Could you check a few things on this model? Use its own coordinates, in mm. Face numbers are marked on the shaded views. Coordinates: 2 decimals unless noted, no trailing zeros. Loops run counter-clockwise (first coordinate to the right, second up) from the corner with the lowest first, then second, coordinate; pieces in that order, holes last. Notation, with made-up numbers: (-9.5, -1.5) - (0.5, -1.5) arc R21 ccw to (0.5, 33.5) - close; hole circle Ø4 at (-25, 59). An arc over 180 degrees is marked (long way). One line per item, written item: value. Start each with the question number.
(1) If I drill on line 1 along X through (y, z) = (-0.7, 0) (3 decimals); line 2 along Z through (x, y) = (0, -0.95) (3 decimals), over which ranges is the centre line in solid material (lowest first)? Write a range as from..to.
(2) If we section it at A-A on z = 0: Write out the boundary of the cut face in (x, y) (3 decimals).
(3) I'm going to push flat-ended pins straight in: P1, Ø1.5, axis at y = -0.5, z = 3, coming from the +X side; P2, Ø2, axis at y = -0.5, z = 8.5, coming from the -X side. Where does each tip first touch, or does it pass through?
(4) If we section it at D-D on y = -1.45: Write out the boundary of the cut face in (x, z) (3 decimals).
(5) If we mould it in two halves opening along X, with no side actions, what happens to the marked faces 1 and 2? For each: pulls with the +X half, pulls with the -X half, needs draft (parallel to the pull), parting line crosses it, or undercut.
(6) If we section it at B-B on x = 0: Write out the boundary of the cut face in (y, z) (3 decimals).
(7) If we section it at C-C on z = 7: Write out the boundary of the cut face in (x, y).
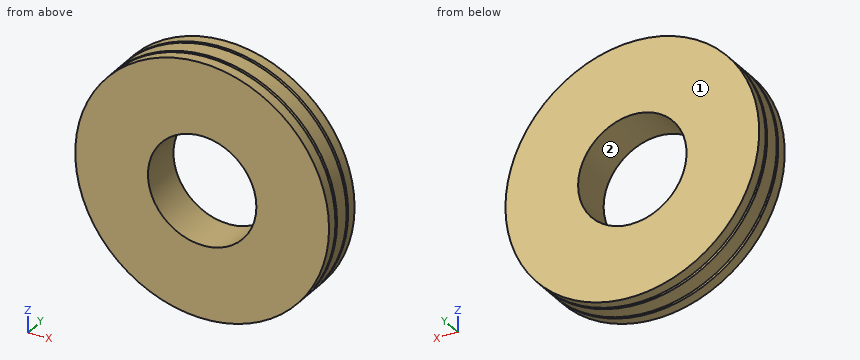
```python
from build123d import *

# Parameters (mm, degrees)
SKETCH1_R           = 11.875
SKETCH1_R_2         = 5.075
BOSS_EXTRUDE1_DEPTH = 2
SKETCH2_R           = 11.875
SKETCH2_R_2         = 11.375
CUT_EXTRUDE1_DEPTH  = 0.25


with BuildPart() as part:
    # Sketch1 → Boss-Extrude1 (new body, symmetric)
    with BuildSketch(Plane(origin=(0, 0, 0), x_dir=(1, 0, 0), z_dir=(0, 1, 0))):
        Circle(SKETCH1_R)
        Circle(SKETCH1_R_2, mode=Mode.SUBTRACT)
    extrude(amount=BOSS_EXTRUDE1_DEPTH, both=True)

    # Sketch2 → Cut-Extrude1 (cut)
    with BuildSketch(Plane(origin=(0, 1, 0), x_dir=(1, 0, 0), z_dir=(0, 1, 0))):
        Circle(SKETCH2_R)
        Circle(SKETCH2_R_2, mode=Mode.SUBTRACT)
    cut_extrude1 = extrude(amount=-CUT_EXTRUDE1_DEPTH, mode=Mode.SUBTRACT)

    # Mirror1: Cut-Extrude1 across plane
    add(cut_extrude1.mirror(Plane.ZX), mode=Mode.SUBTRACT)


solid = part.part
```
Values:
1. line 1: x = -11.875..-5.075, 5.075..11.875
1. line 2: z = -11.375..-5.075, 5.075..11.375
2. outline: (-11.875, -2) - (-5.075, -2) - (-5.075, 2) - (-11.875, 2) - (-11.875, 1) - (-11.375, 1) - (-11.375, 0.75) - (-11.875, 0.75) - (-11.875, -0.75) - (-11.375, -0.75) - (-11.375, -1) - (-11.875, -1) - close; (5.075, -2) - (11.875, -2) - (11.875, -1) - (11.375, -1) - (11.375, -0.75) - (11.875, -0.75) - (11.875, 0.75) - (11.375, 0.75) - (11.375, 1) - (11.875, 1) - (11.875, 2) - (5.075, 2) - close
3. P1: stops at x = 11.66
3. P2: stops at x = -9.21
4. outline: circle Ø23.75 at (0, 0); hole circle Ø10.15 at (0, 0)
5. face 1: needs draft
5. face 2: undercut
6. outline: (-2, -11.875) - (-1, -11.875) - (-1, -11.375) - (-0.75, -11.375) - (-0.75, -11.875) - (0.75, -11.875) - (0.75, -11.375) - (1, -11.375) - (1, -11.875) - (2, -11.875) - (2, -5.075) - (-2, -5.075) - close; (-2, 5.075) - (2, 5.075) - (2, 11.875) - (1, 11.875) - (1, 11.375) - (0.75, 11.375) - (0.75, 11.875) - (-0.75, 11.875) - (-0.75, 11.375) - (-1, 11.375) - (-1, 11.875) - (-2, 11.875) - close
7. outline: (-9.59, -2) - (9.59, -2) - (9.59, -1) - (8.97, -1) - (8.97, -0.75) - (9.59, -0.75) - (9.59, 0.75) - (8.97, 0.75) - (8.97, 1) - (9.59, 1) - (9.59, 2) - (-9.59, 2) - (-9.59, 1) - (-8.97, 1) - (-8.97, 0.75) - (-9.59, 0.75) - (-9.59, -0.75) - (-8.97, -0.75) - (-8.97, -1) - (-9.59, -1) - close
